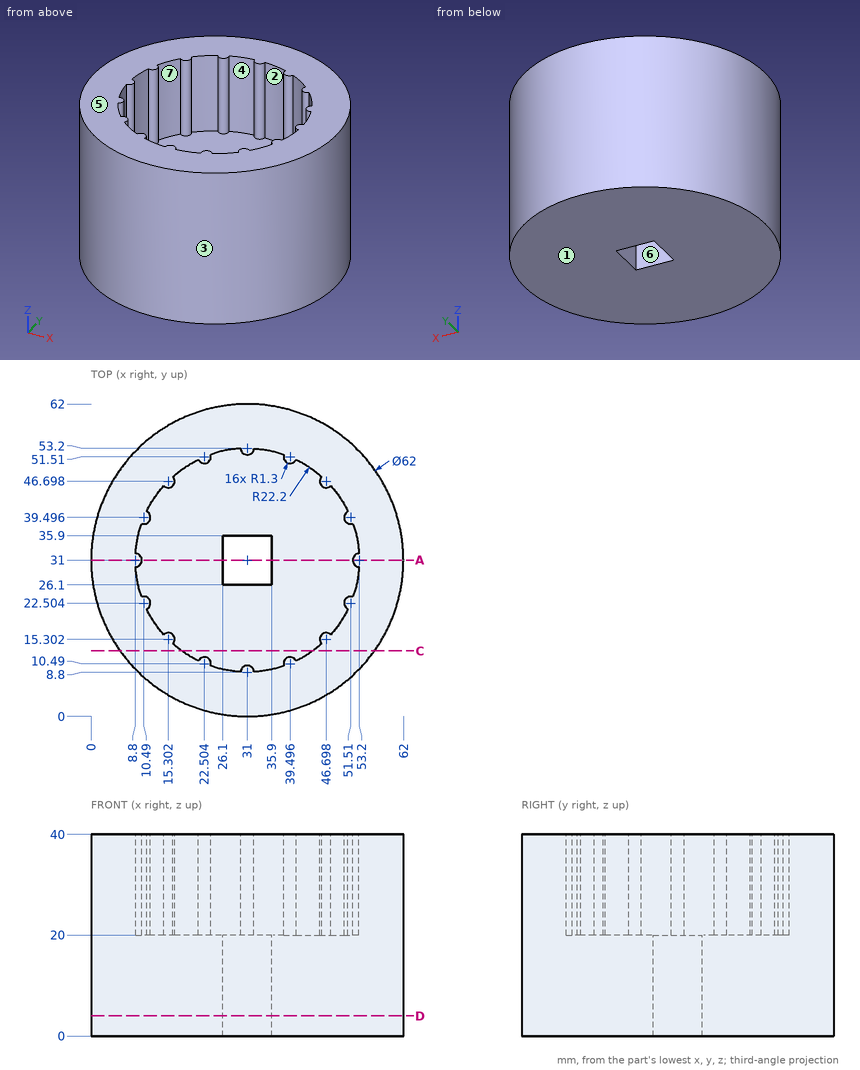
Design review of the part shown in the three views and the two pictorial views. Dimensions are in mm from the part's minimum x, y and z. A direction names the side the tool comes from. Give positions to 0.01 mm unless a question says otherwise; leave off trailing zeros. Write each loop counter-clockwise with the first axis right and the second up, starting at its lowest first coordinate (ties: lowest second). Pieces come first, ordered by that corner, then holes.
Item 1: Machinability: for the marked faces 5, 6 and 7, which of the approach directions +Z, -Z, +X, -X, +Y, -Y give a long, thin tool a straight path to every point of the face, cutting with its end or side? Answer none if there is none.
Item 2: Take a section at D-D (z = 4). Give the boundary of the cut face in (x, y).
Item 3: The part is to be moulded in two halves that separate along X. For the marked faces 1, 2, 3 and 4, say which applies: +X half, -X half, draft (parallel to the pull), parting line (faces both ways), or undercut.
Item 4: Take a section at A-A (y = 31). Give the boundary of the cut face in (x, z).
Item 5: Insertion check: P1, Ø8, axis at x = 30, z = 11, coming from the +Y side; P2, Ø2, axis at x = 14, z = 12, coming from the -Y side; P3, Ø2, axis at x = 33.5, z = 10.5, coming from the -Y side. Each pin has a flat end and moves straight along its axis. Give the tip position at first contact, or say it passes through.
Item 6: Take a section at C-C (y = 13). Give the boundary of the cut face in (x, z), and give its area (3 significant figures).
Item 7: Wall thickness on probe 1 along X at (y, z) = (32, 8); probe 2 along Z at (x, y) = (22, 32.5); probe 3 along Y at (x, z) = (35, 20.5): over which ranges is each line inside the solid? List them lowest first.
Established:
1. face 5: +Z, +X, -X, +Y, -Y
1. face 6: +Z, -Z
1. face 7: +Z
2. outline: circle Ø62 at (31, 31); hole (26.1, 26.1) - (35.9, 26.1) - (35.9, 35.9) - (26.1, 35.9) - close
3. face 1: draft
3. face 2: undercut
3. face 3: parting line
3. face 4: undercut
4. outline: (0, 0) - (26.1, 0) - (26.1, 20) - (10.1, 20) - (10.1, 40) - (0, 40) - close; (35.9, 0) - (62, 0) - (62, 40) - (51.9, 40) - (51.9, 20) - (35.9, 20) - close
5. P1: stops at y = 62
5. P2: stops at y = 4.45
5. P3: stops at y = 0.04
6. outline: (5.76, 0) - (56.24, 0) - (56.24, 40) - (43.99, 40) - (43.99, 20) - (18.01, 20) - (18.01, 40) - (5.76, 40) - close
6. area: 1,500 mm2
7. probe 1: x = 0.02 to 26.1, 35.9 to 61.98
7. probe 2: z = 0 to 20
7. probe 3: y = 0.26 to 9.16, 52.84 to 61.74
